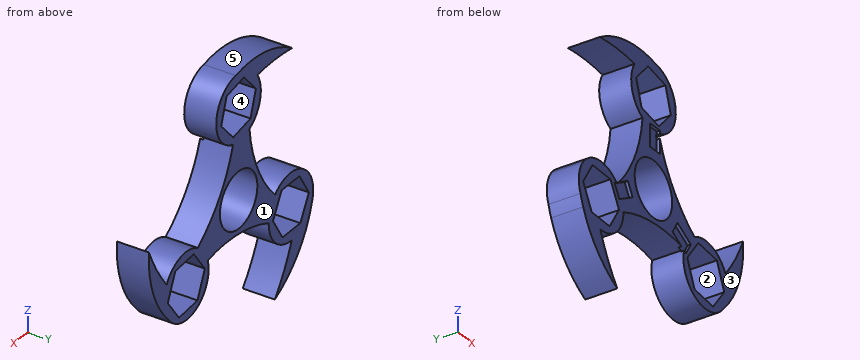
from build123d import *

# Parameters (mm, degrees)
F0_R     = 10.9855
F1_DEPTH = 12.7
F2_W     = 5.655189
F2_H     = 8.981772
F3_DEPTH = 1.27


with BuildPart() as f1:
    # F0 (on Front) → F1 (new body)
    with BuildSketch(Plane.XZ):
        with BuildLine():
            ThreePointArc((-6.360809, 24.00158), (-11.117425, 6.479342), (-21.316083, -8.542029))
            ThreePointArc((-21.316083, -8.542029), (-31.558535, -4.631694), (-41.171763, -9.902784))
            Line((-41.171763, -9.902784), (-41.171763, -17.360528))
            Line((-41.171763, -17.360528), (-35.683101, -8.411922))
            Line((-35.683101, -8.411922), (-25.163529, -8.691618))
            Line((-25.163529, -8.691618), (-20.145967, -17.941683))
            Line((-20.145967, -17.941683), (-25.647977, -26.912052))
            Line((-25.647977, -26.912052), (-36.167549, -26.632355))
            Line((-36.167549, -26.632355), (-41.171763, -17.406898))
            Line((-41.171763, -17.406898), (-41.171763, -27.080146))
            ThreePointArc((-41.171763, -27.080146), (-33.122191, -39.571535), (-21.212272, -48.458844))
            ThreePointArc((-21.212272, -48.458844), (-26.776178, -39.923045), (-31.136971, -30.714332))
            ThreePointArc((-31.136971, -30.714332), (-21.543573, -27.009484), (-17.605574, -17.509412))
            ThreePointArc((-17.605574, -17.509412), (-0.044829, -12.950713), (18.055655, -14.189255))
            ThreePointArc((18.055655, -14.189255), (24.810198, -29.419446), (41.032453, -25.621946))
            ThreePointArc((41.032453, -25.621946), (50.096223, -11.088822), (52.572726, 5.859055))
            ThreePointArc((52.572726, 5.859055), (47.962461, -3.227328), (42.167877, -11.608242))
            ThreePointArc((42.167877, -11.608242), (34.162685, -5.152539), (23.966383, -6.492168))
            ThreePointArc((23.966383, -6.492168), (11.169988, 6.388301), (3.260428, 22.731284))
            ThreePointArc((3.260428, 22.731284), (13.072888, 36.195984), (1.67303, 48.346119))
            ThreePointArc((1.67303, 48.346119), (-15.44491, 48.929013), (-31.360454, 42.599789))
            ThreePointArc((-31.360454, 42.599789), (-21.186282, 43.150373), (-11.030906, 42.322574))
            ThreePointArc((-11.030906, 42.322574), (-12.619113, 32.162023), (-6.360809, 24.00158))
        make_face()
        Circle(F0_R, mode=Mode.SUBTRACT)
        Polygon((37.166687, -8.97331), (41.477768, -19.011964), (34.939579, -27.764796), (24.09031, -26.478974), (19.77923, -16.440321), (26.317418, -7.687489), align=None, mode=Mode.SUBTRACT)
        Polygon((7.046263, 43.085256), (10.207559, 33.166528), (3.198336, 25.469401), (-6.972183, 27.691002), (-10.133479, 37.609731), (-3.124256, 45.306858), align=None, mode=Mode.SUBTRACT)
        with BuildLine():
            Line((-41.171763, -17.360528), (-41.171763, -9.902784))
            ThreePointArc((-41.171763, -9.902784), (-43.63394, -16.110682), (-42.705482, -22.724174))
            ThreePointArc((-42.705482, -22.724174), (-41.998805, -24.92335), (-41.171763, -27.080146))
            Line((-41.171763, -27.080146), (-41.171763, -17.406898))
            Line((-41.171763, -17.406898), (-41.185111, -17.38229))
            Line((-41.185111, -17.38229), (-41.171763, -17.360528))
        make_face()
    extrude(amount=F1_DEPTH)

    # F2 (on face) → F3 (cut)
    with BuildSketch(Plane.XZ.offset(12.7)):
        with Locations((0.939673, 19.659774)):
            Rectangle(F2_W, F2_H)
        Polygon((-22.798719, -8.812781), (-19.971124, -13.710318), (-12.192681, -9.219432), (-15.020276, -4.321895), align=None)
        Polygon((19.031452, -15.337879), (21.859046, -10.440342), (14.080603, -5.949455), (11.253008, -10.846993), align=None)
    extrude(amount=-F3_DEPTH, mode=Mode.SUBTRACT)


solid = f1.part
Can you work these out from the model? Positions are in its coordinate system, mm. Face numbers are marked on the shaded views. A direction names the side the tool comes from. Coordinates: 2 decimals unless noted, no trailing zeros. Write each loop counter-clockwise with the first axis right and the second up, starting at its lowest first coordinate (ties: lowest second). Pieces come first, ordered by that corner, then holes. Notation, with made-up numbers: (41.25, 61.25) - (78.25, 61.25) arc R19 cw to (78.25, 94.25) - close; hole circle Ø2 at (69.25, -36.5). An arc over 180 degrees is marked (long way). Return JSON: item names as keys, results as strings. Group by question number.
Item 1: Which directions (+Z, -Z, +X, -X, +Y, -Y) give clear straight access to the entire face, cutting with the end or side of a thin tool? Please do the marked faces 1 and 2.
Item 2: If we section it at B-B (z = 30.5): Write out the boundary of the cut face in (x, y), then the cut area to 3 significant figures.
Item 3: If we section it at A-A (x = 38.5): Write out the boundary of the cut face in (y, z).
Item 4: If we section it at D-D (z = -21): Write out the boundary of the cut face in (x, y).
Item 5: I'm going to push flat-ended pins straight in: pin 1 Ø4.5 at (x, z) = (-18.5, -9) entering from -Y; pin 2 Ø0.6 at (x, y) = (0, -12) entering from +Z; pin 3 Ø0.6 at (y, z) = (-12, 17) entering from -X; pin 4 Ø7.5 at (x, z) = (18.5, -9.5) entering from -Y. Where does each tip first touch, or does it pass through?
Item 6: Please list where these lines run through material, in increasing order: probe 1 along Z at (x, y) = (0, -3); probe 2 along Z at (x, y) = (-29, -11.5); probe 3 along X at (y, z) = (-9, 3).
Item 7: We'd pull the mould along Z, two halves only. Please class the marked faces 3, 4 and 5: pulls with the +Z half, pulls with the -Z half, needs draft (parallel to the pull), parting line crosses it, or undercut.
Item 8: If we section it at C-C (x = 0): Write out the boundary of the cut face in (y, z), then the cut area to 3 significant figures.
Return value:
{
 "1": {"face 1": "+Z, -Z, +X, -X, +Y", "face 2": "+Y, -Y"},
 "2": {"outline": "(-12.07, -12.7) - (-7.87, -12.7) - (-7.87, 0) - (-12.07, 0) - close; (7.78, -12.7) - (12.15, -12.7) - (12.15, 0) - (7.78, 0) - close", "area": "109 mm^2"},
 "3": {"outline": "(-12.7, -28.15) - (0, -28.15) - (0, -23) - (-12.7, -23) - close; (-12.7, -12.08) - (0, -12.08) - (0, -7.3) - (-12.7, -7.3) - close"},
 "4": {"outline": "(-43.29, -12.7) - (-39.22, -12.7) - (-39.22, 0) - (-43.29, 0) - close; (-22.02, -12.7) - (-18.04, -12.7) - (-18.04, 0) - (-22.02, 0) - close; (17.98, -12.7) - (21.74, -12.7) - (21.74, 0) - (17.98, 0) - close; (39.99, -12.7) - (44.86, -12.7) - (44.86, 0) - (39.99, 0) - close"},
 "5": {"pin 1": "stops at y = -11.43", "pin 2": "stops at z = 48.78", "pin 3": "stops at x = -7.59", "pin 4": "stops at y = -12.7"},
 "6": {"probe 1": "z = -12.95 to -10.99, 10.99 to 26.17, 44.62 to 48.72", "probe 2": "z = -43.43 to -35.63, -30.62 to -26.82, -8.59 to -4.71, 42.85 to 44.05", "probe 3": "x = -12.87 to -10.57, 10.57 to 13.77, 51.29 to 52.65"},
 "7": {"face 3": "needs draft", "face 4": "undercut", "face 5": "pulls with the +Z half"},
 "8": {"outline": "(-12.7, -12.95) - (0, -12.95) - (0, -10.99) - (-12.7, -10.99) - close; (-12.7, 10.99) - (0, 10.99) - (0, 26.17) - (-12.7, 26.17) - (-12.7, 24.15) - (-11.43, 24.15) - (-11.43, 15.17) - (-12.7, 15.17) - close; (-12.7, 44.62) - (0, 44.62) - (0, 48.72) - (-12.7, 48.72) - close", "area": "258 mm^2"}
}
